```python
from build123d import *

# Parameters (mm, degrees)
F0_W     = 76.2
F0_H     = 38.1
F1_DEPTH = 20.32
F2_W     = 63.5
F2_H     = 6.35
F3_DEPTH = 13.97
F4_W     = 17.78
F4_H     = 6.35
F5_DEPTH = 5.588


with BuildPart() as f1:
    # F0 (on Top) → F1 (new body)
    with BuildSketch(Plane.XY):
        Rectangle(F0_W, F0_H)
    extrude(amount=F1_DEPTH)

    # F2 (on face) → F3 (cut)
    with BuildSketch(Plane(origin=(0, 0, 0), x_dir=(1, 0, 0), z_dir=(0, 0, -1))):
        Polygon((-31.75, -12.7), (-31.75, 12.7), (-31.75, 19.05), (-38.1, 19.05), (-38.1, -19.05), (-31.75, -19.05), align=None)
        with Locations((0, 15.875)):
            Rectangle(F2_W, F2_H)
        Polygon((31.75, 19.05), (31.75, 12.7), (31.75, -12.7), (31.75, -19.05), (38.1, -19.05), (38.1, 19.05), align=None)
        with Locations((0, -15.875)):
            Rectangle(F2_W, F2_H)
    extrude(amount=-F3_DEPTH, mode=Mode.SUBTRACT)

    # F4 (on face) → F5 (cut)
    with BuildSketch(Plane.XY.offset(20.32)):
        with Locations((23.13825, 12.661981)):
            Rectangle(F4_W, F4_H)
        with Locations((23.13825, 6.311981)):
            Rectangle(F4_W, F4_H)
        with Locations((23.13825, -4.518458)):
            Rectangle(F4_W, F4_H)
        with Locations((23.13825, -10.868458)):
            Rectangle(F4_W, F4_H)
        with Locations((0, -10.868458)):
            Rectangle(F4_W, F4_H)
        with Locations((0, -4.518458)):
            Rectangle(F4_W, F4_H)
        with Locations((-24.402459, -10.868458)):
            Rectangle(F4_W, F4_H)
        with Locations((-24.402459, -4.518458)):
            Rectangle(F4_W, F4_H)
        with Locations((-24.085267, 6.311981)):
            Rectangle(F4_W, F4_H)
        with Locations((-24.085267, 12.661981)):
            Rectangle(F4_W, F4_H)
        with Locations((0, 12.661981)):
            Rectangle(F4_W, F4_H)
        with Locations((0, 6.311981)):
            Rectangle(F4_W, F4_H)
    extrude(amount=-F5_DEPTH, mode=Mode.SUBTRACT)


solid = f1.part
```
Input: part model. Units: mm. Frame: model coordinates. A direction names the side the tool comes from. Round coordinates to 2 decimals unless told otherwise and drop trailing zeros. Loops run counter-clockwise (first coordinate to the right, second up) from the corner with the lowest first, then second, coordinate; pieces in that order, holes last. Notation, with made-up numbers: (40.25, -36.75) - (75.25, -36.75) arc R13 cw to (75.25, -18.75) - close; hole circle Ø3 at (18.25, 55). An arc over 180 degrees is marked (long way). One line per item, written item: value. Start each with the question number.
(1) Section C-C, the plane z = 10.5. Return loops of the section in (x, y).
(2) Section D-D, the plane x = -10. Return loops of the section in (y, z).
(3) Section B-B, the plane y = 7. Return loops of the section in (x, z), plus the area to 3 significant figures.
(4) Draft query along X for faces 1 (the flat face through (-25, -1.343, 18)), 2 (the flat face through (-31.75, 0, 7)), 3 (the flat face through (38.1, 0, 17)), 4 (the flat face through (0, 12.7, 7)). Return one class per face: +X half, -X half, draft (parallel to the pull), parting line (faces both ways), or undercut.
(5) Access query for faces 5 (the flat face through (-25, -8, 14.732)), 6 (the flat face through (0, -12.7, 7)). Directions: +Z, -Z, +X, -X, +Y, -Y. A direction counts if a zero-diameter tool reaches every point of the face in a straight line with its end or side. Return the directions, or none.
(6) Ray query, line 1 (X direction, y = -7, z = 18); line 2 (Y direction, x = -23, z = 19); line 3 (Z direction, x = 4, y = 14). Return the intervals inside material, ascending. Write a range as [from, to].
(7) Section A-A, the plane x = -18. Return loops of the section in (y, z).
(8) Contact query for flat-ended pins moving along their axis: P1, Ø11, axis at x = 8.5, z = 9, coming from the -Y side; P2, Ø5, axis at y = -6, z = 3, coming from the -X side; P3, Ø1, axis at x = -21, y = -7.5, coming from the +Z side; P4, Ø3, axis at x = 29, z = 5.5, coming from the +Y side. Output: stop coordinate, or through.
Results below:
1. outline: (-31.75, -12.7) - (31.75, -12.7) - (31.75, 12.7) - (-31.75, 12.7) - close
2. outline: (-19.05, 13.97) - (-12.7, 13.97) - (-12.7, 0) - (12.7, 0) - (12.7, 13.97) - (19.05, 13.97) - (19.05, 20.32) - (-19.05, 20.32) - close
3. outline: (-38.1, 13.97) - (-31.75, 13.97) - (-31.75, 0) - (31.75, 0) - (31.75, 13.97) - (38.1, 13.97) - (38.1, 20.32) - (32.03, 20.32) - (32.03, 14.73) - (14.25, 14.73) - (14.25, 20.32) - (8.89, 20.32) - (8.89, 14.73) - (-8.89, 14.73) - (-8.89, 20.32) - (-15.2, 20.32) - (-15.2, 14.73) - (-32.98, 14.73) - (-32.98, 20.32) - (-38.1, 20.32) - close
3. area: 1,070 mm^2
4. face 1: undercut
4. face 2: -X half
4. face 3: +X half
4. face 4: draft
5. face 5: +Z
5. face 6: -Z, +X, -X, -Y
6. line 1: [-38.1, -33.29], [-15.51, -8.89], [8.89, 14.25], [32.03, 38.1]
6. line 2: [-19.05, -14.04], [-1.34, 3.14], [15.84, 19.05]
6. line 3: [13.97, 14.73]
7. outline: (-19.05, 13.97) - (-12.7, 13.97) - (-12.7, 0) - (12.7, 0) - (12.7, 13.97) - (19.05, 13.97) - (19.05, 20.32) - (15.84, 20.32) - (15.84, 14.73) - (3.14, 14.73) - (3.14, 20.32) - (-1.34, 20.32) - (-1.34, 14.73) - (-14.04, 14.73) - (-14.04, 20.32) - (-19.05, 20.32) - close
8. P1: y = -19.05
8. P2: x = -31.75
8. P3: z = 14.73
8. P4: y = 12.7
